from build123d import *

# Parameters (mm, degrees)
CUT_EXTRUDE_THIN1_START = -65.5
CUT_EXTRUDE_THIN1_DEPTH = 65.5


# Read off the part's stored shape, not the designer's step: Cut-Extrude-Thin1
with BuildPart() as part:
    # Sketch3 → Revolve1 (revolve)
    with BuildSketch(Plane.XY, mode=Mode.PRIVATE) as revolve1_sk:
        Polygon((-38, 55), (-38, 70.548970685), (-29, 70.548970685), (-29, 55), (-29, 0), (-31.5, 0), (-41.9, 55), align=None)
    revolve(revolve1_sk.sketch.rotate(Axis((0, 0, 0), (0, 1, 0)), 270), axis=Axis((0, 0, 0), (0, 1, 0)))

    # Cut-Extrude-Thin1 outline → Cut-Extrude-Thin1 (cut)
    with BuildSketch(Plane(origin=(0, 70.548970685, 0), x_dir=(1, 0, 0), z_dir=(0, 1, 0)).offset(CUT_EXTRUDE_THIN1_START)):
        Polygon((2.875, 4.979646072), (2.875, 43), (-2.875, 43), (-2.875, 4.979646072), (0, 3.319764048), align=None)
        Polygon((5.75, 0), (2.875, -1.659882024), (2.875, -4.979646072), (23.55351401, -16.918391702), (34.763443099, -23.390447279), (37.551270189, -25), (39, -25), (39, -19.19689645), (37.638443099, -18.410801207), (26.42851401, -11.93874563), align=None)
        Polygon((-2.875, -4.979646072), (-2.875, -1.659882024), (-5.75, 0), (-26.42851401, -11.93874563), (-37.638443099, -18.410801207), (-39, -19.19689645), (-39, -25), (-37.551270189, -25), (-34.763443099, -23.390447279), (-23.55351401, -16.918391702), align=None)
    extrude(amount=CUT_EXTRUDE_THIN1_DEPTH, mode=Mode.SUBTRACT)


solid = part.part
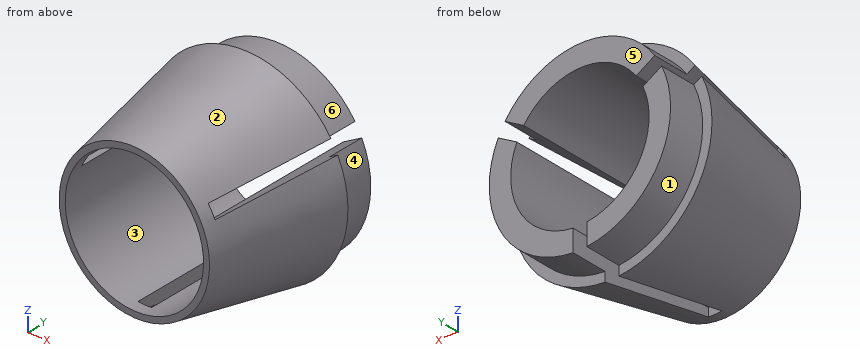
Could you check a few things on this model? Use its own coordinates, in mm. Face numbers are marked on the shaded views. A direction names the side the tool comes from. Give positions to 0.01 mm unless a question says otherwise; leave off trailing zeros. Loops run counter-clockwise (first coordinate to the right, second up) from the corner with the lowest first, then second, coordinate; pieces in that order, holes last. Notation, with made-up numbers: (59.5, -25) -> (103.5, -25) arc R22 ccw to (103.5, 3) -> close; hole circle Ø3 at (-17, 43). An arc over 180 degrees is marked (long way). Return JSON: item names as keys, results as strings.
Item 1: If we section it at D-D on y = 60: List the corners of the cut face in (x, z) for me (3 decimals), plus the area to 3 significant figures.
Geometry results:
{"outline": "(-34.252, 16.456) arc R38 ccw to (-2.875, -37.891) -> (-2.875, -28.857) arc R29 cw to (-26.429, 11.939) -> close; (-31.377, 21.435) -> (-23.554, 16.918) arc R29 cw to (23.554, 16.918) -> (31.377, 21.435) arc R38 ccw to start; (2.875, -37.891) arc R38 ccw to (34.252, 16.456) -> (26.429, 11.939) arc R29 cw to (2.875, -28.857) -> close", "area": "1,740 mm²"}
Item 2: If we section it at A-A on z = 0: List the corners of the cut face in (x, y) for me, plus the area to 3 significant figures.
Geometry results:
{"outline": "(-41.9, 55) -> (-31.5, 0) -> (-29, 0) -> (-29, 70.55) -> (-38, 70.55) -> (-38, 55) -> close; (29, 0) -> (31.5, 0) -> (41.9, 55) -> (38, 55) -> (38, 70.55) -> (29, 70.55) -> close", "area": "1,130 mm²"}
Item 3: If we section it at B-B on y = 33.5: List the corners of the cut face in (x, z) for me (3 decimals), plus the area to 3 significant figures.
Geometry results:
{"outline": "(-34.108, 16.373) arc R37.835 ccw to (-2.875, -37.725) -> (-2.875, -28.857) arc R29 cw to (-26.429, 11.939) -> close; (-31.233, 21.352) -> (-23.554, 16.918) arc R29 cw to (23.554, 16.918) -> (31.233, 21.352) arc R37.835 ccw to start; (2.875, -37.725) arc R37.835 ccw to (34.108, 16.373) -> (26.429, 11.939) arc R29 cw to (2.875, -28.857) -> close", "area": "1,700 mm²"}
Item 4: We'd pull the mould along X, two halves only. Please class the marked faces 3, 4, 5 and 6: +X half, -X half, draft (parallel to the pull), parting line (faces both ways), or undercut.
Geometry results:
{"face 3": "undercut", "face 4": "+X half", "face 5": "draft", "face 6": "parting line"}
Item 5: If we section it at C-C on x = 0: List the corners of the cut face in (y, z) for me.
Geometry results:
{"outline": "(0, -31.5) -> (5.05, -32.45) -> (5.05, -29) -> (0, -29) -> close; (0, 29) -> (70.55, 29) -> (70.55, 38) -> (55, 38) -> (55, 41.9) -> (0, 31.5) -> close"}
Item 6: I'm going to push flat-ended pins straight in: pin 1 (1.8 mm diameter, centred on x = -0.5, z = -31.5, fed in from +Y); pin 2 (14 mm diameter, centred on y = 45.5, z = -38, fed in from -X); pin 3 (10.5 mm diameter, centred on y = 37.5, z = -33.5, fed in from +X); pin 4 (5 mm diameter, centred on x = 17.5, z = -16.5, fed in from +Y). Where does each tip first touch, or does it pass through?
Geometry results:
{"pin 1": "stops at y = 5.05", "pin 2": "stops at x = -25.69", "pin 3": "stops at x = 26.48", "pin 4": "passes through"}
Item 7: Which directions (+Z, -Z, +X, -X, +Y, -Y) give clear straight access to the entire face, cutting with the end or side of a thin tool? Please do the marked faces 1 and 2.
Geometry results:
{"face 1": "-X, +Y", "face 2": "-Y"}
Item 8: I need wall thicknesses on L1, parallel to Z at x = -26.5, y = 38; L2, parallel to Z at x = -16, y = 30.5; L3, parallel to Z at x = 6, y = 30. Which ranges of each line are inside material? Lowest first, please. Write a range as from..to.
Geometry results:
{"L1": "z = -28.18..-11.78, 11.78..11.98, 18.62..28.18", "L2": "z = -33.66..-24.19, 24.19..33.66", "L3": "z = -36.69..-28.37, 28.37..36.69"}
